Source: CAD feature listing. Evaluate the final solid. Frame: model axes, mm. A direction names the side the tool comes from. Give positions to 0.01 mm unless a question says otherwise; leave off trailing zeros. Loops run counter-clockwise (first coordinate to the right, second up) from the corner with the lowest first, then second, coordinate; pieces in that order, holes last. Notation, with made-up numbers: M 45,3 L 82,3 A7 cw 82,16 Z; hole C 81,89.25 d6. An arc over 180 degrees is marked long. Put each result on its own line as item: value.
from build123d import *

# Parameters (mm, degrees)
SKETCH1_R           = 28
SKETCH1_R_2         = 16
BOSS_EXTRUDE1_DEPTH = 16
SKETCH2_R           = 15
SKETCH2_R_2         = 9
BOSS_EXTRUDE2_DEPTH = 10
BOSS_EXTRUDE3_DEPTH = 4
BOSS_EXTRUDE4_DEPTH = 4
BOSS_EXTRUDE5_DEPTH = 60
CUT_EXTRUDE1_DEPTH  = 216.77207691
HOLE1_D             = 5
HOLE1_CBORE_D       = 12
HOLE1_CBORE_DEPTH   = 6
BOSS_EXTRUDE6_START = 2
SKETCH9_R           = 7.5
SKETCH9_R_2         = 2.5
BOSS_EXTRUDE6_DEPTH = 2
FILLET1_R           = 30
FILLET2_R           = 2


with BuildPart() as part:
    # Sketch1 → Boss-Extrude1 (new, symmetric)
    with BuildSketch(Plane.XY):
        Circle(SKETCH1_R)
        Circle(SKETCH1_R_2, mode=Mode.SUBTRACT)
    extrude(amount=BOSS_EXTRUDE1_DEPTH, both=True)



with BuildPart() as body_2:
    # Sketch2 → Boss-Extrude2 (new, symmetric)
    with BuildSketch(Plane.XY):
        with Locations((-72, 0)):
            Circle(SKETCH2_R)
        with Locations((-72, 0)):
            Circle(SKETCH2_R_2, mode=Mode.SUBTRACT)
    extrude(amount=BOSS_EXTRUDE2_DEPTH, both=True)


with BuildPart() as part_1:
    add(part.part)

    add(body_2.part)  # Boss-Extrude3 merges body 2
    # Sketch3 → Boss-Extrude3 (add, symmetric)
    with BuildSketch(Plane.XY):
        with BuildLine():
            Line((-72, 15), (-5.155280446, 27.521320527))
            ThreePointArc((-5.155280446, 27.521320527), (-28, 0), (-5.155280446, -27.521320527))
            Line((-5.155280446, -27.521320527), (-72, -15))
            ThreePointArc((-72, -15), (-57, 0), (-72, 15))
        make_face()
    extrude(amount=BOSS_EXTRUDE3_DEPTH, both=True)

    # Sketch4 → Boss-Extrude4 (add, symmetric)
    with BuildSketch(Plane.XY):
        with BuildLine():
            Line((70.070865753, 81.750068946), (86.438826394, 64.197580107))
            Line((86.438826394, 64.197580107), (25.1229929, -12.362654559))
            ThreePointArc((25.1229929, -12.362654559), (22.301575109, 16.930438496), (-5.155280446, 27.521320527))
            Line((-5.155280446, 27.521320527), (-10.933902304, 26.438871876))
            Line((-10.933902304, 26.438871876), (70.070865753, 81.750068946))
        make_face()
    extrude(amount=BOSS_EXTRUDE4_DEPTH, both=True)

    # Sketch5 → Boss-Extrude5 (add)
    with BuildSketch(Plane(origin=(0, 0, -4), x_dir=(-1, 0, 0), z_dir=(0, 0, -1))):
        Polygon((-70.070865753, 81.750068946), (-81.041171277, 91.980044347), (-97.409131918, 74.427555508), (-86.438826394, 64.197580107), align=None)
    extrude(amount=-BOSS_EXTRUDE5_DEPTH)

    # Sketch6 → Cut-Extrude1 (cut, through all)
    with BuildSketch(Plane(origin=(89.225151598, 83.203799928, 0), x_dir=(0, 0, -1), z_dir=(0.7313537016191697, 0.6819983600624995, 0))):
        with BuildLine():
            Line((-56, 12), (-56, 0))
            ThreePointArc((-56, 0), (-52.485281374, 8.485281374), (-44, 12))
            Line((-44, 12), (-56, 12))
        make_face()
        with BuildLine():
            Line((-56, 0), (-56, -12))
            Line((-56, -12), (-44, -12))
            ThreePointArc((-44, -12), (-52.485281374, -8.485281374), (-56, 0))
        make_face()
    extrude(amount=-CUT_EXTRUDE1_DEPTH, mode=Mode.SUBTRACT)

    # Hole1 (through all)
    with Locations(Plane(origin=(78.254846073, 72.973824527, 0), x_dir=(0, 0, 1), z_dir=(-0.7313537016191697, -0.6819983600624995, 0))):
        with Locations((44, 0)):
            CounterBoreHole(HOLE1_D / 2, HOLE1_CBORE_D / 2, HOLE1_CBORE_DEPTH)

    # Sketch9 → Boss-Extrude6 (add)
    with BuildSketch(Plane(origin=(89.225151598, 83.203799928, 0), x_dir=(0, 0, -1), z_dir=(0.7313537016191697, 0.6819983600624995, 0)).offset(BOSS_EXTRUDE6_START)):
        with Locations(Location((-44, 0, 0), (0, 0, 90))):
            Circle(SKETCH9_R)
        with Locations(Location((-44, 0, 0), (0, 0, 270))):
            Circle(SKETCH9_R_2, mode=Mode.SUBTRACT)
    extrude(amount=-BOSS_EXTRUDE6_DEPTH)

    # Fillet1
    fillet1_edges = [part_1.edges().sort_by_distance(p)[0] for p in [
        (-10.933902304, 26.438871876, 0),
    ]]
    fillet(fillet1_edges, radius=FILLET1_R)

    # Fillet2
    fillet2_edges = [part_1.edges().sort_by_distance(p)[0] for p in [
        (94.340139298, 77.718647165, 44),
    ]]
    fillet(fillet2_edges, radius=FILLET2_R - 0.0001)  # a hair under: the kernel refuses the full size


solid = part_1.part
1. Section query A-A (z = 7.5). Output: boundary loops of the cut face in (x, y), plus the area to 3 significant figures.
Found:
outline: C -72,0 d30; C 0,0 d56; M 70.07,81.75 L 86.44,64.2 L 97.41,74.43 L 81.04,91.98 Z; hole C -72,0 d18; hole C 0,0 d32
area: 2,470 mm^2
2. Material intervals for line 1 (X direction, y = 1.5, z = -8); line 2 (Y direction, x = 13.5, z = 6.5); line 3 (Z direction, x = -30, y = -12.5), sorted ascending. Write a range as from..to.
Found:
line 1: -86.92..-80.87, -63.13..-57.08, -27.96..-15.93, 15.93..27.96
line 2: -24.53..-8.59, 8.59..24.53
line 3: -4..4
3. Section query C-C (x = 0). Output: boundary loops of the cut face in (y, z).
Found:
outline: M -28,-16 L -16,-16 L -16,16 L -28,16 Z; M 16,-16 L 28,-16 L 28,-4 L 33.9,-4 L 33.9,4 L 28,4 L 28,16 L 16,16 Z
4. Section query B-B (y = -7). Output: boundary loops of the cut face in (x, z).
Found:
outline: M -85.27,-10 L -77.66,-10 L -77.66,10 L -85.27,10 Z; M -66.34,-10 L -58.73,-10 L -58.73,-4 L -27.11,-4 L -27.11,-16 L -14.39,-16 L -14.39,16 L -27.11,16 L -27.11,4 L -58.73,4 L -58.73,10 L -66.34,10 Z; M 14.39,-16 L 27.11,-16 L 27.11,-4 L 29.42,-4 L 29.42,4 L 27.11,4 L 27.11,16 L 14.39,16 Z
5. Section query D-D (x = -70). Output: boundary loops of the cut face in (y, z).
Found:
outline: M -15.37,-4 L -14.87,-4 L -14.87,-10 L -8.77,-10 L -8.77,10 L -14.87,10 L -14.87,4 L -15.37,4 Z; M 8.77,-10 L 14.87,-10 L 14.87,-4 L 15.37,-4 L 15.37,4 L 14.87,4 L 14.87,10 L 8.77,10 Z
6. Contact query for flat-ended pins moving along their axis: P1, Ø23.5, axis at x = -72, y = 0, coming from the +Z side; P2, Ø10, axis at x = 8.5, z = 15, coming from the -Y side; P3, Ø17, axis at x = -13.5, y = -4.5, coming from the +Z side. Output: stop coordinate, or through.
Found:
P1: z = 10
P2: y = -27.78
P3: z = 16
7. Access query for faces 1 (the flat face through (-65.5, -6.5, -10)), 2 (the flat face through (78.37, 72.85, 29.64)), 3 (the cylindrical face through (12.92, -24.84, 0.22)). Directions: +Z, -Z, +X, -X, +Y, -Y. A direction counts if a zero-diameter tool reaches every point of the face in a straight line with its end or side. Return the directions, or none.
Found:
face 1: -Z, -X, +Y, -Y
face 2: +Z, -X, -Y
face 3: none
